The model under review builds one solid part; all positions refer to its coordinate system, in mm. Face numbers are marked on the shaded views. A direction names the side the tool comes from. Give positions to 0.01 mm unless a question says otherwise; leave off trailing zeros. Write each loop counter-clockwise with the first axis right and the second up, starting at its lowest first coordinate (ties: lowest second). Pieces come first, ordered by that corner, then holes. Notation, with made-up numbers: M 61.5,54.25 L 100.5,54.25 A20 ccw 100.5,68.25 Z; hole C -31,85.25 d1. An arc over 180 degrees is marked long. Write item = value, one per line. Start each with the question number.
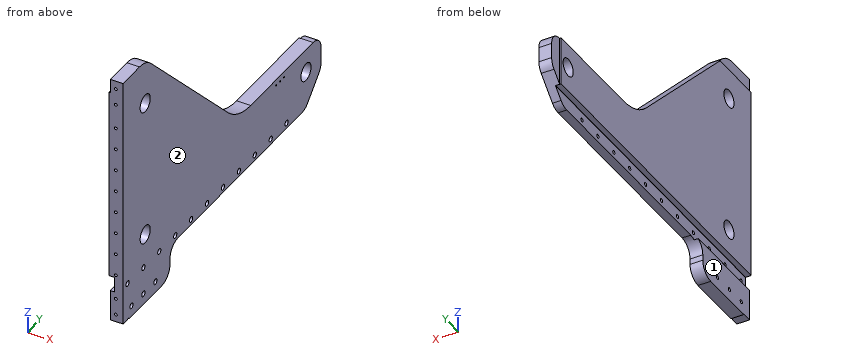
```python
from build123d import *

# Parameters (mm, degrees)
BOSS_EXTRUDE1_DEPTH                                  = 50.8
SKETCH2_W                                            = 20
SKETCH2_H                                            = 55
CUT_EXTRUDE1_DEPTH                                   = 1485.951393144
SKETCH3_W                                            = 50.8
SKETCH3_H                                            = 5
CUT_EXTRUDE2_DEPTH                                   = 1553.894278436
SKETCH5_W                                            = 115
SKETCH5_H                                            = 323.205505282
CUT_EXTRUDE5_DEPTH                                   = 5
M6_TAPPED_HOLE1_D                                    = 5
M6_TAPPED_HOLE1_DEPTH                                = 20
M6_TAPPED_HOLE1_TIP                                  = 1.502151548
CBORE_FOR_M12_HEX_SOCKET_HEAD_CAP_SCREW1_D           = 13.5
CBORE_FOR_M12_HEX_SOCKET_HEAD_CAP_SCREW1_CBORE_D     = 20
CBORE_FOR_M12_HEX_SOCKET_HEAD_CAP_SCREW1_CBORE_DEPTH = 13
M12_TAPPED_HOLE1_D                                   = 10.2
M12_TAPPED_HOLE1_DEPTH                               = 43.99
M12_TAPPED_HOLE1_TIP                                 = 3.064389157
FILLET1_R                                            = 0.79375
SKETCH14_W                                           = 225
SKETCH14_H                                           = 50.8
SKETCH14_W_2                                         = 50.8
SKETCH14_H_2                                         = 195.8
CUT_EXTRUDE6_DEPTH                                   = 1485.788752654
SKETCH15_R                                           = 31.75
SKETCH15_W                                           = 3.175
SKETCH15_H                                           = 38.1
CUT_EXTRUDE7_DEPTH                                   = 1485.951393147
SKETCH16_R                                           = 31.75
CUT_EXTRUDE8_DEPTH                                   = 1485.951393144


with BuildPart() as part:
    # Sketch1 → Boss-Extrude1 (new body)
    with BuildSketch(Plane(origin=(0, 0, 0), x_dir=(0, 0, -1), z_dir=(1, 0, 0))):
        with BuildLine():
            Line((0, 350), (0, 1129.289321881))
            ThreePointArc((0, 1129.289321881), (-3.806023374, 1148.4234935), (-14.644660941, 1164.644660941))
            Line((-14.644660941, 1164.644660941), (-85.355339059, 1235.355339059))
            ThreePointArc((-85.355339059, 1235.355339059), (-101.5765065, 1246.193976626), (-120.710678119, 1250))
            Line((-120.710678119, 1250), (-175, 1250))
            ThreePointArc((-175, 1250), (-210.355339059, 1235.355339059), (-225, 1200))
            Line((-225, 1200), (-225, 807.842712475))
            ThreePointArc((-225, 807.842712475), (-240.224093498, 731.306026002), (-283.578643763, 666.421356237))
            Line((-283.578643763, 666.421356237), (-770.710678119, 179.289321881))
            ThreePointArc((-770.710678119, 179.289321881), (-792.387953251, 146.846986999), (-800, 108.578643763))
            Line((-800, 108.578643763), (-800, 0))
            Line((-800, 0), (0, 0))
            Line((0, 0), (120, 0))
            Line((120, 0), (120, 250))
            ThreePointArc((120, 250), (105.355339059, 285.355339059), (70, 300))
            Line((70, 300), (50, 300))
            ThreePointArc((50, 300), (14.644660941, 314.644660941), (0, 350))
        make_face()
    extrude(amount=BOSS_EXTRUDE1_DEPTH)

    # Sketch2 → Cut-Extrude1 (cut, through all)
    with BuildSketch(Plane(origin=(0, 1250, 0), x_dir=(1, 0, 0), z_dir=(0, 1, 0))):
        with Locations((10, -22.5)):
            Rectangle(SKETCH2_W, SKETCH2_H)
    extrude(amount=-CUT_EXTRUDE1_DEPTH, mode=Mode.SUBTRACT)

    # Sketch3 → Cut-Extrude2 (cut, through all)
    with BuildSketch(Plane(origin=(0, 0, 800), x_dir=(-1, 0, 0), z_dir=(0, 0, -1))):
        with Locations((-25.4, 2.5)):
            Rectangle(SKETCH3_W, SKETCH3_H)
    extrude(amount=CUT_EXTRUDE2_DEPTH, mode=Mode.SUBTRACT)

    # Sketch5 → Cut-Extrude5 (cut)
    with BuildSketch(Plane(origin=(0, 0, 0), x_dir=(0, 0, -1), z_dir=(1, 0, 0))):
        with Locations((62.5, 166.602752641)):
            Rectangle(SKETCH5_W, SKETCH5_H)
    extrude(amount=CUT_EXTRUDE5_DEPTH, mode=Mode.SUBTRACT)

    # M6 Tapped Hole1
    with Locations(Plane(origin=(50.8, 0, 0), x_dir=(0, 0, -1), z_dir=(1, 0, 0))):
        with Locations((-204, 1017), (-204, 967), (-204, 992)):
            Hole(M6_TAPPED_HOLE1_D / 2, depth=M6_TAPPED_HOLE1_DEPTH)
            with Locations((0, 0, -(M6_TAPPED_HOLE1_DEPTH + M6_TAPPED_HOLE1_TIP / 2))):  # 118° drill point
                Cone(0, M6_TAPPED_HOLE1_D / 2, M6_TAPPED_HOLE1_TIP, mode=Mode.SUBTRACT)

    # CBORE for M12 Hex Socket Head Cap Screw1 (through all)
    with Locations(Plane(origin=(50.8, 0, 0), x_dir=(0, 0, -1), z_dir=(1, 0, 0))):
        with Locations((-20, 33), (-20, 133), (-20, 233), (-20, 333), (-20, 433), (-20, 533), (-20, 633), (-20, 733), (-20, 833), (-20, 933), (-20, 1033), (80, 58), (80, 133), (80, 208)):
            CounterBoreHole(CBORE_FOR_M12_HEX_SOCKET_HEAD_CAP_SCREW1_D / 2, CBORE_FOR_M12_HEX_SOCKET_HEAD_CAP_SCREW1_CBORE_D / 2, CBORE_FOR_M12_HEX_SOCKET_HEAD_CAP_SCREW1_CBORE_DEPTH)

    # M12 Tapped Hole1
    with Locations(Plane(origin=(0, 5, 0), x_dir=(-1, 0, 0), z_dir=(0, -1, 0))):
        with Locations((-25, -770), (-25, 90), (-25, 30), (-25, -60), (-25, -140), (-25, -220), (-25, -300), (-25, -380), (-25, -460), (-25, -540), (-25, -620), (-25, -710)):
            Hole(M12_TAPPED_HOLE1_D / 2, depth=M12_TAPPED_HOLE1_DEPTH)
            with Locations((0, 0, -(M12_TAPPED_HOLE1_DEPTH + M12_TAPPED_HOLE1_TIP / 2))):  # 118° drill point
                Cone(0, M12_TAPPED_HOLE1_D / 2, M12_TAPPED_HOLE1_TIP, mode=Mode.SUBTRACT)

    # Fillet1
    fillet1_edges = [part.edges().sort_by_distance(p)[0] for p in [
        (20, 602.5, 50),
        (20, 166.602752641, -5),
    ]]
    fillet(fillet1_edges, radius=FILLET1_R)

    # Sketch14 → Cut-Extrude6 (cut, through all)
    with BuildSketch(Plane.ZY.offset(-5)):
        with Locations((112.5, 1224.6)):
            Rectangle(SKETCH14_W, SKETCH14_H)
        with Locations((774.6, 102.9)):
            Rectangle(SKETCH14_W_2, SKETCH14_H_2)
    extrude(amount=CUT_EXTRUDE6_DEPTH, mode=Mode.SUBTRACT)

    # Sketch15 → Cut-Extrude7 (cut, through all)
    with BuildSketch(Plane.ZY):
        with Locations((139.6896, 144.2936)):
            Circle(SKETCH15_R)
        with Locations((-118.4125, 24.05)):
            Rectangle(SKETCH15_W, SKETCH15_H)
    extrude(amount=-CUT_EXTRUDE7_DEPTH, mode=Mode.SUBTRACT)

    # Sketch16 → Cut-Extrude8 (cut, through all)
    with BuildSketch(Plane(origin=(50.8, 0, 0), x_dir=(0, 0, -1), z_dir=(1, 0, 0))):
        with Locations((-139.6896, 1155)):
            Circle(SKETCH16_R)
        with Locations((-639.6896, 144.2936)):
            Circle(SKETCH16_R)
    extrude(amount=-CUT_EXTRUDE8_DEPTH, mode=Mode.SUBTRACT)


solid = part.part
```
Item 1: We need section A-A, the plane y = 365.5. Write out the cut boundary in (x, z), and give its area (3 significant figures).
Item 2: Clearance check with flat-ended pins moving along their axes: P1, Ø1, axis at y = 628, z = 30, coming from the -X side; P2, Ø11, axis at y = 333, z = 20, coming from the -X side; P3, Ø10, axis at x = 13, y = 791, coming from the +Z side; P4, Ø3, axis at x = 45.5, z = 435, coming from the +Y side. State where each tip first meets the part, or that it passes through.
Item 3: To check wall thickness, follow probe 1 along Z at (x, y) = (34.25, 1033); probe 2 along Z at (x, y) = (2.5, 173); probe 3 along Z at (x, y) = (35.5, 59). State the ranges of each line that lie inside material, in increasing order. Write a range as [from, to].
Item 4: For the marked faces 1 and 2, list the 3-axis set-ups (+Z, -Z, +X, -X, +Y, -Y) from which the entire face can be reached by the end or side of a thin tool; tool diameter is ignored.
Worked out:
q1.outline = M 0,50 L 19.21,50 A0.79 cw 20,49.21 L 20,0 L 50.8,0 L 50.8,584.5 L 0,584.5 Z
q1.area = 28,700 mm²
q2.P1 = 20
q2.P2 = through
q2.P3 = 226.2
q2.P4 = 516.5
q3.probe_1 = [0, 13.25], [26.75, 225]
q3.probe_2 = [50, 126.12], [153.25, 626.12], [653.25, 749.2]
q3.probe_3 = [-120, -86.68], [-73.32, 800]
q4.face_1 = -Z, -X, +Y, -Y
q4.face_2 = +Z, -Z, +X, +Y, -Y
